Verification items for the finished model (mm, model axes). A direction names the side the tool comes from. Round coordinates to 2 decimals unless told otherwise and drop trailing zeros. Loops run counter-clockwise (first coordinate to the right, second up) from the corner with the lowest first, then second, coordinate; pieces in that order, holes last. Notation, with made-up numbers: M 72,75.5 L 126,75.5 A15 ccw 126,80.5 Z; hole C 61.25,63 d4. An arc over 180 degrees is marked long. Answer as CSV lines item,"result".
Autodesk Inventor part; units mm, degrees
ref_plane "Work Plane1" through (33.575, 0, 0) normal (0, 0, -1) x (1, 0, 0)
ref_plane "YZ Plane" through (0, 0, 0) normal (1, 0, 0) x (0, 1, 0)
ref_plane "XZ Plane" through (0, 0, 0) normal (0, 1, 0) x (-1, 0, 0)
sketch "Эскиз1" plane through (0, 0, 0) normal (0, 0, 1) x (1, 0, 0)
  line L0 (0, 0) -> (16, 0)
  line L1 (16, 0) -> (16, 4)
  line L2 (16, 4) -> (5.25, 4)
  line L3 (5.25, 4) -> (4.4832, 4)
  line L4 (4.4832, 4) -> (4, 4)
  line L5 (4, 4) -> (0.75, 7.25)
  line L6 (0.75, 7.25) -> (0, 7.25)
  line L7 (0, 7.25) -> (0, 0)
  line L8 (5.25, 4) -> (4, 4) construction
  line L9 (-3.2, 0) -> (19.2, 0)
  line L10 (0, 8.7) -> (0, -1.45)
  point P0 (4, 4)
  dimension "d0" = 16
  dimension "d1" = 45
  dimension "d2" = 0.7668
  dimension "d3" = 10.75
  dimension "d4" = 4
  dimension "d5" = 8
  dimension "d6" = 8
  dimension "d7" = 14.5
revolve "Базовый элемент" add sketch "Эскиз1" angle 360 about axis through (0, 0, 0) along (1, 0, 0)
sketch "Эскиз2" plane through (0, 0, 0) normal (-1, 0, 0) x (0, 0, 1)
  line L0 (0.5375, 7.25) -> (0.5375, -7.25)
  line L1 (0.5375, -7.25) -> (-0.5375, -7.25)
  line L2 (-0.5375, -7.25) -> (-0.5375, 7.25)
  line L3 (-0.5375, 7.25) -> (0.5375, 7.25)
  line L4 (-0.5375, 0) -> (0.5375, 0) construction
  line L5 (0, -7.25) -> (0, 7.25) construction
  line L6 (0, 7.25) -> (0, 0)
  dimension "d15" = 1.075
  dimension "d16" = 14.5
extrude "Паз" cut sketch "Эскиз2" against normal blind 2.2
thread "Резьба"
ref_plane "Work Plane1" through (33.575, 0, 0) normal (0, 0, -1) x (1, 0, 0)
chamfer "Фаска2" distance 1.6 angle 45 1 edges at (16, -4, 0)
equation "\"d0\" = NLG"
equation "\"d2\" = GAL"
equation "\"d3\" = GEL"
equation "\"d5\" = BDM"
equation "\"d6\" = GD"
equation "\"d15\" = SBR"
equation "\"d16\" = KOD"
equation "\"NLG\" = 16"
equation "\"GAL\" = 0.61345 * PTC"
equation "\"GEL\" = 10.75"
equation "\"KOH\" = 4"
equation "\"KOD\" = 14.5"
equation "\"SEWI\" = 90deg"
equation "\"BDM\" = NND"
equation "\"GD\" = NND"
equation "\"SBR\" = 1.075"
equation "\"STI\" = 3.8"
equation "\"SPD\" = NND - 1.2269 * PTC"
equation "\"GUL\" = 0.61345 * PTC"
equation "\"PTC\" = 1.25"
equation "\"EPV\" = 8"
equation "\"THREADDIA\" = 8"
equation "\"TOA\" = 30deg"
equation "\"FAWI\" = 45deg"
equation "\"RR\" = 0.1 * NND"
equation "\"NND\" = 8"
equation "\"GD1\" = THREADDIA - 1.2269 * PTC"
properties part number "Винт M8-6gx16 ГОСТ 17475-80" material "Сталь, мягкая"
1) Go/stop test with flat-tipped pins: pin 1 (4 mm diameter, centred on y = 1.5, z = 4.5, fed in from +X); pin 2 (1 mm diameter, centred on x = 6, z = 1, fed in from +Y); pin 3 (1 mm diameter, centred on y = -3.5, z = -3.5, fed in from +X). Record where each tip stops, or that it passes through.
Here are the results:
pin 1,"stops at x = 15.66"
pin 2,"stops at y = 3.97"
pin 3,"stops at x = 3.55"
2) Draft check along Z on faces 4 (the flat face through (0, 0, 3)), 5 (the cylindrical face through (0.37, 0.15, -7.25)), 6 (the flat face through (2.2, 0, 0)), 7 (the flat face through (1, 0, 0.538)). Enter one of: +Z half, -Z half, draft (parallel to the pull), parting line (faces both ways), or undercut.
Here are the results:
face 4,"draft"
face 5,"-Z half"
face 6,"undercut"
face 7,"undercut"
3) Section check C-C (x = 7). Record the cut outline in (y, z), plus the area to 3 significant figures.
Here are the results:
outline,"C 0,0 d8"
area,"50.3 mm^2"
4) Material ranges on probe 1 along Z at (x, y) = (11.75, 0); probe 2 along Z at (x, y) = (7.5, -1.5); probe 3 along X at (y, z) = (1.75, 0), recorded low to high.
Here are the results:
probe 1,"z = -4 to 4"
probe 2,"z = -3.71 to 3.71"
probe 3,"x = 2.2 to 16"
5) Section check B-B (y = 0). Record the cut outline in (x, z).
Here are the results:
outline,"M 0,-7.25 L 0.75,-7.25 L 4,-4 L 14.4,-4 L 16,-2.4 L 16,2.4 L 14.4,4 L 4,4 L 0.75,7.25 L 0,7.25 L 0,0.54 L 2.2,0.54 L 2.2,-0.54 L 0,-0.54 Z"
6) Section check A-A (z = 0). Record the cut outline in (x, y), plus the area to 3 significant figures.
Here are the results:
outline,"M 2.2,-5.8 L 4,-4 L 14.4,-4 L 16,-2.4 L 16,2.4 L 14.4,4 L 4,4 L 2.2,5.8 Z"
area,"111 mm^2"
7) Set-up check for faces 1 (the cylindrical face through (9.127, -0.867, 3.905)), 2 (the flat face through (1, 0, -0.538)), 3 (the cylindrical face through (0.37, -0.15, 7.25)): record each of +Z, -Z, +X, -X, +Y, -Y from which the full face is reachable in a straight line by a thin tool's end or side.
Here are the results:
face 1,"+X"
face 2,"-X, +Y, -Y"
face 3,"+Z, +X, -X"
8) Section check D-D (x = 3.5). Record the cut outline in (y, z).
Here are the results:
outline,"C 0,0 d9"
